Work out the finished part from the listing and answer in its coordinate system (mm). A direction names the side the tool comes from. Coordinates: 2 decimals unless noted, no trailing zeros. Write each loop counter-clockwise with the first axis right and the second up, starting at its lowest first coordinate (ties: lowest second). Pieces come first, ordered by that corner, then holes. Notation, with made-up numbers: (9.25, 47) - (17.25, 47) arc R15 cw to (17.25, 54) - close; hole circle Ø3 at (77, -19.75). An arc over 180 degrees is marked (long way). One line per item, written item: value.
```python
from build123d import *

# Parameters (mm, degrees)
SKETCH1_W           = 50
SKETCH1_H           = 34
BOSS_EXTRUDE1_DEPTH = 3
SKETCH2_W           = 38
SKETCH2_H           = 34
BOSS_EXTRUDE2_DEPTH = 3
SKETCH3_R           = 1.25
CUT_EXTRUDE1_DEPTH  = 3
BOSS_EXTRUDE3_DEPTH = 34
CUT_EXTRUDE4_DEPTH  = 43.626282972
SKETCH6_W           = 7
SKETCH6_H           = 4.004114793
CUT_EXTRUDE3_DEPTH  = 54.150729064
FILLET1_R           = 0.2
SKETCH8_W           = 4.910344877
SKETCH8_H           = 2.364797993
CUT_EXTRUDE5_DEPTH  = 43.626282972
FILLET2_R           = 0.5
SKETCH9_W           = 50
SKETCH9_H           = 6.499651724
CUT_EXTRUDE6_DEPTH  = 43.626282972
CHAMFER1_START      = -18
CHAMFER1_DEPTH      = 36


with BuildPart() as part:
    # Sketch1 → Boss-Extrude1 (new body)
    with BuildSketch(Plane(origin=(0, 0, 0), x_dir=(1, 0, 0), z_dir=(0, 1, 0))):
        Rectangle(SKETCH1_W, SKETCH1_H)
    extrude(amount=BOSS_EXTRUDE1_DEPTH)

    # Sketch2 → Boss-Extrude2 (add)
    with BuildSketch(Plane(origin=(0, 3, 0), x_dir=(1, 0, 0), z_dir=(0, 1, 0))):
        Rectangle(SKETCH2_W, SKETCH2_H)
    extrude(amount=BOSS_EXTRUDE2_DEPTH)

    # Sketch3 → Cut-Extrude1 (cut)
    with BuildSketch(Plane(origin=(0, 3, 0), x_dir=(1, 0, 0), z_dir=(0, 1, 0))):
        with Locations(Location((22, 8, 0), (0, 0, 270))):
            Circle(SKETCH3_R)
        with Locations(Location((22, -8, 0), (0, 0, 90))):
            Circle(SKETCH3_R)
        with Locations(Location((-22, -8, 0), (0, 0, 270))):
            Circle(SKETCH3_R)
        with Locations(Location((-22, 8, 0), (0, 0, 90))):
            Circle(SKETCH3_R)
    extrude(amount=-CUT_EXTRUDE1_DEPTH, mode=Mode.SUBTRACT)

    # Sketch5 → Boss-Extrude3 (add)
    with BuildSketch(Plane.XY.offset(17)):
        with BuildLine():
            Line((10.162882175, 0), (-10.162882175, 0))
            ThreePointArc((-10.162882175, 0), (-5.40902103, -3.588814383), (-0.175438596, -0.74480324))
            ThreePointArc((-0.175438596, -0.74480324), (0, -0.640830834), (0.175438596, -0.74480324))
            ThreePointArc((0.175438596, -0.74480324), (5.40902103, -3.588814383), (10.162882175, 0))
        make_face()
    extrude(amount=-BOSS_EXTRUDE3_DEPTH)

    # Sketch7 → Cut-Extrude4 (cut, through all)
    with BuildSketch(Plane(origin=(0, 0, -17), x_dir=(-1, 0, 0), z_dir=(0, 0, -1))):
        with BuildLine():
            Line((-8.541784002, 2.785692228), (-8.541784002, 8.770064047))
            Line((-8.541784002, 8.770064047), (8.249387021, 8.770064047))
            Line((8.249387021, 8.770064047), (8.249387021, 2.975059658))
            ThreePointArc((8.249387021, 2.975059658), (5.18491916, -0.185254174), (2.049991811, 2.905179016))
            Line((2.049991811, 2.905179016), (2.049991811, 5.195476311))
            Line((2.049991811, 5.195476311), (-2.343419325, 5.195476311))
            Line((-2.343419325, 5.195476311), (-2.343419325, 2.855696601))
            ThreePointArc((-2.343419325, 2.855696601), (-5.40689232, -0.341101373), (-8.541784002, 2.785692228))
        make_face()
    extrude(amount=-CUT_EXTRUDE4_DEPTH, mode=Mode.SUBTRACT)

    # Sketch6 → Cut-Extrude3 (cut, through all)
    with BuildSketch(Plane(origin=(25, 0, 0), x_dir=(0, 0, -1), z_dir=(1, 0, 0))):
        with Locations((0, -2.578040121)):
            Rectangle(SKETCH6_W, SKETCH6_H)
    extrude(amount=-CUT_EXTRUDE3_DEPTH, mode=Mode.SUBTRACT)

    # Fillet1
    fillet1_edges = [part.edges().sort_by_distance(p)[0] for p in [
        (10.162882175, 0, 0),
        (-10.162882175, 0, 0),
    ]]
    fillet(fillet1_edges, radius=FILLET1_R)

    # Sketch8 → Cut-Extrude5 (cut, through all)
    with BuildSketch(Plane(origin=(0, 0, -17), x_dir=(-1, 0, 0), z_dir=(0, 0, -1))):
        with Locations((-0.118869912, 4.00385134)):
            Rectangle(SKETCH8_W, SKETCH8_H)
    extrude(amount=-CUT_EXTRUDE5_DEPTH, mode=Mode.SUBTRACT)


with BuildPart() as cut_extrude5_kept_piece:
    # of the separate pieces the step leaves, the one the design keeps (cut_extrude5_pieces_kept)
    add(part.part.solids().sort_by_distance((-10.300657517, 0, -17))[0])

    # Fillet2
    fillet2_edges = [cut_extrude5_kept_piece.edges().sort_by_distance(p)[0] for p in [
        (8.541784002, 6, 0),
        (-8.249387021, 6, 0),
    ]]
    fillet(fillet2_edges, radius=FILLET2_R)

    # Sketch9 → Cut-Extrude6 (cut, through all)
    with BuildSketch(Plane(origin=(0, 0, -17), x_dir=(-1, 0, 0), z_dir=(0, 0, -1))):
        with Locations((0, 6.036788854)):
            Rectangle(SKETCH9_W, SKETCH9_H)
    extrude(amount=-CUT_EXTRUDE6_DEPTH, mode=Mode.SUBTRACT)

    # Chamfer1: read off the stored shape, not the designer's step
    # Chamfer1 outline → Chamfer1 (cut)
    with BuildSketch(Plane.XY.offset(CHAMFER1_START)):
        with BuildLine():
            ThreePointArc((8.541784002, 2.785692228), (8.541581007, 2.714125068), (8.539725958, 2.642581666))
            Line((8.539725958, 2.642581666), (8.689620689, 2.786962992))
            Line((8.689620689, 2.786962992), (8.541784002, 2.786962992))
            Line((8.541784002, 2.786962992), (8.541784002, 2.785692228))
        make_face()
        with BuildLine():
            Line((2.342030341, 2.786962992), (2.192030341, 2.786962992))
            Line((2.192030341, 2.786962992), (2.344386261, 2.634607072))
            ThreePointArc((2.344386261, 2.634607072), (2.342272067, 2.710770555), (2.342030341, 2.786962992))
        make_face()
        with BuildLine():
            ThreePointArc((-2.052604274, 2.786962992), (-2.05696798, 2.706483589), (-2.063422436, 2.62614483))
            Line((-2.063422436, 2.62614483), (-1.902604274, 2.786962992))
            Line((-1.902604274, 2.786962992), (-2.052604274, 2.786962992))
        make_face()
        with BuildLine():
            Line((-8.397351028, 2.786962992), (-8.236532866, 2.62614483))
            ThreePointArc((-8.236532866, 2.62614483), (-8.242987322, 2.706483589), (-8.247351028, 2.786962992))
            Line((-8.247351028, 2.786962992), (-8.397351028, 2.786962992))
        make_face()
    extrude(amount=CHAMFER1_DEPTH, mode=Mode.SUBTRACT)


solid = cut_extrude5_kept_piece.part
```
Item 1: Section C-C, the plane y = 1.75 is taken. Determine the outline of the cut face in (x, z).
Evaluation:
outline: (-25, -17) - (-8.02, -17) - (-8.02, 17) - (-25, 17) - close; (-2.28, -17) - (2.51, -17) - (2.51, 17) - (-2.28, 17) - close; (8.37, -17) - (25, -17) - (25, 17) - (8.37, 17) - close; hole circle Ø2.5 at (-22, -8); hole circle Ø2.5 at (-22, 8); hole circle Ø2.5 at (22, -8); hole circle Ø2.5 at (22, 8)
Item 2: Which of the six approach directions +Z, -Z, +X, -X, +Y, -Y give full straight-line access (tool end or side, diameter ignored) to faces 1 (the face through (18, 0, 0)), 2 (the face through (5.25, -3.6, 4.02)), 3 (the face through (-2, -2, 3.5)), 4 (the face through (-18, 0, 0))?
Evaluation:
face 1: +Z, -Z, +X, -Y
face 2: +Z, -Z, -Y
face 3: +X, -X, -Y
face 4: +Z, -Z, -X, -Y
Item 3: Consider probe 1 along Z at (x, y) = (-8, -1); probe 2 along X at (y, z) = (1.5, -8); probe 3 along X at (y, z) = (0.5, 4.5). Determine where each line is inside the solid, lowest interval first.
Evaluation:
probe 1: z = -17 to -3.5, 3.5 to 17
probe 2: x = -25 to -23.25, -20.75 to -7.91, -2.39 to 2.61, 8.27 to 20.75, 23.25 to 25
probe 3: x = -25 to -7.09, -3.21 to 3.32, 7.57 to 25
Item 4: Section D-D, the plane y = -3 is taken. Determine the outline of the cut face in (x, z).
Evaluation:
outline: (-7.51, -17) - (-2.49, -17) - (-2.49, -3.5) - (-7.51, -3.5) - close; (-7.51, 3.5) - (-2.49, 3.5) - (-2.49, 17) - (-7.51, 17) - close; (2.49, -17) - (7.51, -17) - (7.51, -3.5) - (2.49, -3.5) - close; (2.49, 3.5) - (7.51, 3.5) - (7.51, 17) - (2.49, 17) - close
Item 5: Section B-B, the plane z = 8 is taken. Determine the outline of the cut face in (x, y).
Evaluation:
outline: (-25, 0) - (-23.25, 0) - (-23.25, 2.79) - (-25, 2.79) - close; (-20.75, 0) - (-10.3, 0) arc R0.2 cw to (-10.11, -0.13) arc R5.5 ccw to (-0.18, -0.74) arc R0.2 cw to (0.18, -0.74) arc R5.5 ccw to (10.11, -0.13) arc R0.2 cw to (10.3, 0) - (20.75, 0) - (20.75, 2.79) - (8.69, 2.79) - (8.54, 2.64) arc R3.1 cw to (2.34, 2.63) - (2.19, 2.79) - (-1.9, 2.79) - (-2.06, 2.63) arc R3.1 cw to (-8.24, 2.63) - (-8.4, 2.79) - (-20.75, 2.79) - close; (23.25, 0) - (25, 0) - (25, 2.79) - (23.25, 2.79) - close
Item 6: Given pin 1 (4.5 mm diameter, centred on x = 19, z = -6.5, fed in from -Y); pin 2 (2 mm diameter, centred on x = -1.5, z = 0.5, fed in from -Y), each flat-ended and moving along its own axis, determine where each tip first touches the part or whether it passes through.
Evaluation:
pin 1: stops at y = 0
pin 2: stops at y = -0.58
Item 7: Section A-A, the plane x = 22 is taken. Determine the outline of the cut face in (y, z), then the cut area to 3 significant figures.
Evaluation:
outline: (0, -17) - (2.79, -17) - (2.79, -9.25) - (0, -9.25) - close; (0, -6.75) - (2.79, -6.75) - (2.79, 6.75) - (0, 6.75) - close; (0, 9.25) - (2.79, 9.25) - (2.79, 17) - (0, 17) - close
area: 80.8 mm2
Item 8: Determine the mould class of faces 5 (the face through (23.22, 1.41, 8.27)), 6 (the face through (0, 0, 17)), 7 (the face through (-25, 1, 0)), 8 (the face through (-5.428, -3.587, 4.016)) for opening direction X: +X half, -X half, draft (parallel to the pull), parting line (faces both ways), or undercut.
Evaluation:
face 5: undercut
face 6: draft
face 7: -X half
face 8: undercut
